Geometry check sheet. Reference: drawing and pictorial views, mm from the part's lowest x, y, z. A direction names the side the tool comes from. Round coordinates to 2 decimals unless told otherwise and drop trailing zeros. Order: outer loops, then holes, each group sorted by start corner. A loop starts at its lowest first (then second) coordinate and runs counter-clockwise, first axis right, second up. Notation, with made-up numbers: M 87,-11 L 99,-11 A26 cw 99,13 Z; hole C 7,-28 d3. An arc over 180 degrees is marked long. Answer as a JSON object with one key per item and string values. Group by question number.
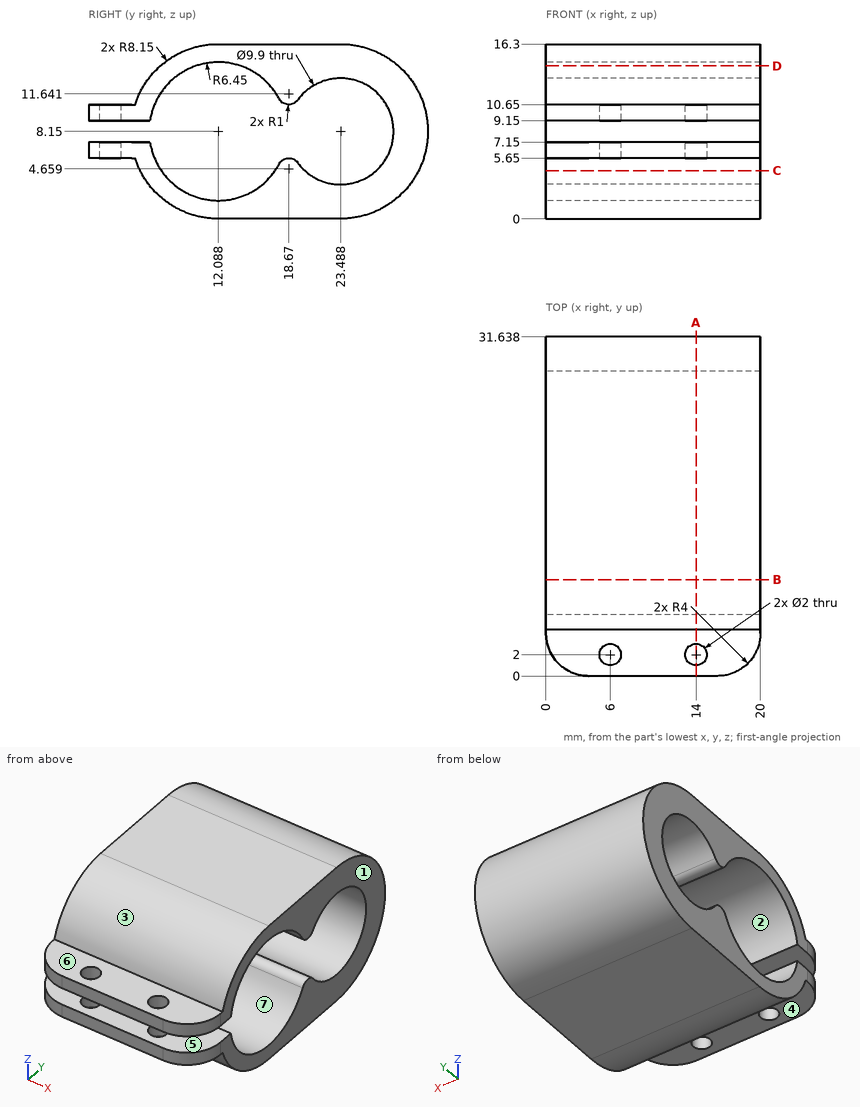
Q1. Gauge pin test, flat ends, axial feed: pin 1 Ø1 at (y, z) = (6.5, 6.5) entering from +X; pin 2 Ø3 at (x, y) = (6, 2) entering from +Z; pin 3 Ø2 at (x, z) = (17, 4.5) entering from -Y; pin 4 Ø6.5 at (x, y) = (5, 4) entering from +Z. Record the tip position at first contact, or that the pin passes through.
Q2. Cross-section at A-A, the plane x = 14. Record the cut outline in (y, z).
Q3. Thickness scan on line 1 (Y direction, x = 15.5, z = 10.75) (1 decimal); line 2 (Y direction, x = 1.75, z = 11) (1 decimal); line 3 (Z direction, x = 9, y = 3). Record the ranges inside material, lowest first. Write a range as from..to.
Q4. Release check for a two-part mould opening along Z. For the marked faces 1, 2 and 3 record: released by +Z, released by -Z, zero draft, split by the parting line, or undercut.
Q5. Cross-section at C-C, the plane z = 4.5. Record the cut outline in (x, y) (1 decimal).
Q6. Tool access check on the marked faces 4, 5, 6 and 7. Record the directions out of +Z, -Z, +X, -X, +Y, -Y that give a thin tool (end or side, any length) a straight path to the whole face; none if there is none.
Q7. Cross-section at B-B, the plane y = 9. Record the cut outline in (x, z).
Q8. Cross-section at D-D, the plane z = 14.25. Record the cut outline in (x, y) (1 decimal), then the cut area to 3 significant figures.
Conclusion:
{
 "1": {"pin 1": "through", "pin 2": "z = 10.65", "pin 3": "y = 4.38", "pin 4": "z = 14.71"},
 "2": {"outline": "M 0,5.65 L 1,5.65 L 1,7.15 L 0,7.15 Z; M 0,9.15 L 1,9.15 L 1,10.65 L 0,10.65 Z; M 3,5.65 L 4.33,5.65 A8.15 ccw 12.09,0 L 23.49,0 A8.15 ccw 23.49,16.3 L 12.09,16.3 A8.15 ccw 4.33,10.65 L 3,10.65 L 3,9.15 L 5.72,9.15 A6.45 cw 17.79,11.17 A1 ccw 19.48,11.05 A4.95 cw long 19.48,5.25 A1 ccw 17.79,5.13 A6.45 cw 5.72,7.15 L 3,7.15 Z"},
 "3": {"line 1": "4.4..6.2, 18.2..19.1, 27.7..31.2", "line 2": "4.5..6.3, 17.9..19.4, 27.5..31.1", "line 3": "5.65..7.15, 9.15..10.65"},
 "4": {"face 1": "zero draft", "face 2": "undercut", "face 3": "released by +Z"},
 "5": {"outline": "M 0,4.8 L 20,4.8 L 20,6.8 L 0,6.8 Z; M 0,17.4 L 20,17.4 L 20,20.1 L 0,20.1 Z; M 0,26.8 L 20,26.8 L 20,30.8 L 0,30.8 Z"},
 "6": {"face 4": "-Z, +X, -X, -Y", "face 5": "+X, -X, -Y", "face 6": "+Z, +X, -X, -Y", "face 7": "+X, -X"},
 "7": {"outline": "M 0,0.61 L 20,0.61 L 20,2.49 L 0,2.49 Z; M 0,13.81 L 20,13.81 L 20,15.69 L 0,15.69 Z"},
 "8": {"outline": "M 0,6.7 L 20,6.7 L 20,10 L 0,10 Z; M 0,14.2 L 20,14.2 L 20,28.9 L 0,28.9 Z", "area": "360 mm2"}
}
